Work out the finished part from the listing and answer in its coordinate system (mm). A direction names the side the tool comes from. Round coordinates to 2 decimals unless told otherwise and drop trailing zeros. Order: outer loops, then holes, each group sorted by start corner. A loop starts at its lowest first (then second) coordinate and runs counter-clockwise, first axis right, second up. Notation, with made-up numbers: (67.5, 3.25) -> (93.5, 3.25) arc R20 cw to (93.5, 33.25) -> close; hole circle Ø5 at (87.5, 9.25). An arc over 180 degrees is marked (long way). Use one line per item in the form item = value.
```python
from build123d import *

# Parameters (mm, degrees)
SKETCH2_R               = 18
BOSS_EXTRUDE1_DEPTH     = 22
SKETCH3_R               = 18.5
BOSS_EXTRUDE2_DEPTH     = 26.5
SKETCH4_R               = 1.5
CUT_EXTRUDE1_DEPTH      = 6
CIRPATTERN1_COUNT       = 6
SKETCH5_R               = 6
BOSS_EXTRUDE3_DEPTH     = 6
SKETCH6_R               = 3
BOSS_EXTRUDE4_DEPTH     = 15.5
CUT_EXTRUDE2_DEPTH      = 1
CUT_EXTRUDE2_DEPTH_BACK = 12


with BuildPart() as part:
    # Sketch2 → Boss-Extrude1 (new body)
    with BuildSketch(Plane(origin=(0, 0, 0), x_dir=(1, 0, 0), z_dir=(0, 1, 0))):
        Circle(SKETCH2_R)
    extrude(amount=BOSS_EXTRUDE1_DEPTH)

    # Sketch3 → Boss-Extrude2 (add)
    with BuildSketch(Plane(origin=(0, 22, 0), x_dir=(1, 0, 0), z_dir=(0, 1, 0))):
        Circle(SKETCH3_R)
    extrude(amount=BOSS_EXTRUDE2_DEPTH)

    # Sketch4 → Cut-Extrude1 (cut)
    with BuildSketch(Plane(origin=(0, 48.5, 0), x_dir=(1, 0, 0), z_dir=(0, 1, 0))):
        with Locations((-15.5, 0)):
            Circle(SKETCH4_R)
    cut_extrude1 = extrude(amount=-CUT_EXTRUDE1_DEPTH, mode=Mode.SUBTRACT)

    # CirPattern1: Cut-Extrude1 ×6 about axis
    cirpattern1_axis = Axis((0, 0, 0), (0, 1, 0))
    for i in range(1, CIRPATTERN1_COUNT):
        add(cut_extrude1.rotate(cirpattern1_axis, i * 360 / CIRPATTERN1_COUNT), mode=Mode.SUBTRACT)

    # Sketch5 → Boss-Extrude3 (add)
    with BuildSketch(Plane(origin=(0, 48.5, 0), x_dir=(1, 0, 0), z_dir=(0, 1, 0))):
        with Locations((0, 7)):
            Circle(SKETCH5_R)
    extrude(amount=BOSS_EXTRUDE3_DEPTH)

    # Sketch6 → Boss-Extrude4 (add)
    with BuildSketch(Plane(origin=(0, 54.5, 0), x_dir=(1, 0, 0), z_dir=(0, 1, 0))):
        with Locations((0, 7)):
            Circle(SKETCH6_R)
    extrude(amount=BOSS_EXTRUDE4_DEPTH)

    # Sketch7 → Cut-Extrude2 (cut, two sides)
    with BuildSketch(Plane(origin=(0, 70, 0), x_dir=(1, 0, 0), z_dir=(0, 1, 0))) as cut_extrude2_sk:
        Polygon((-80.661403086, 9.5), (-1.6583, 9.5), (1.6583, 9.5), (80.661403086, 9.5), (80.661403086, 167.506206173), (-80.661403086, 167.506206173), align=None)
    extrude(amount=CUT_EXTRUDE2_DEPTH, mode=Mode.SUBTRACT)
    extrude(cut_extrude2_sk.sketch, amount=-CUT_EXTRUDE2_DEPTH_BACK, mode=Mode.SUBTRACT)


solid = part.part
```
Item 1: The part is cut by section B-B, the plane z = 0. Give the vertices of the cut face in (x, y).
Findings:
outline = (-18.5, 22) -> (-18, 22) -> (-18, 0) -> (18, 0) -> (18, 22) -> (18.5, 22) -> (18.5, 48.5) -> (17, 48.5) -> (17, 42.5) -> (14, 42.5) -> (14, 48.5) -> (-14, 48.5) -> (-14, 42.5) -> (-17, 42.5) -> (-17, 48.5) -> (-18.5, 48.5) -> close
Item 2: The part is cut by section D-D, the plane z = 5. Give the vertices of the cut face in (x, y), and give its area (3 significant figures).
Findings:
outline = (-17.81, 22) -> (-17.29, 22) -> (-17.29, 0) -> (17.29, 0) -> (17.29, 22) -> (17.81, 22) -> (17.81, 48.5) -> (-17.81, 48.5) -> close
area = 1,700 mm^2
Item 3: Consider line 1 along Z through (x, y) = (-7.75, 44); line 2 along Y through (x, z) = (7, 9); line 3 along Y through (x, z) = (-12, -14). Determine where each line is inside the solid, lowest interval first.
Findings:
line_1 = -16.8 to -14.92, -11.92 to 11.92, 14.92 to 16.8
line_2 = 0 to 48.5
line_3 = 22 to 48.5
Item 4: Determine the mould class of faces 6 (the cylindrical face through (17, 46, 0)), 7 (the cylindrical face through (-0.78, 51.46, -12.95)), 8 (the flat face through (4.02, 22, 17.73)) for opening direction X: released by +X, released by -X, zero draft, split by the parting line, or undercut.
Findings:
face_6 = undercut
face_7 = split by the parting line
face_8 = zero draft
Item 5: The part is cut by section A-A, the plane x = 0. Give the vertices of the cut face in (y, z), and give its area (3 significant figures).
Findings:
outline = (0, -18) -> (22, -18) -> (22, -18.5) -> (48.5, -18.5) -> (48.5, -13) -> (54.5, -13) -> (54.5, -10) -> (58, -10) -> (58, -9.5) -> (70, -9.5) -> (70, -4) -> (54.5, -4) -> (54.5, -1) -> (48.5, -1) -> (48.5, 18.5) -> (22, 18.5) -> (22, 18) -> (0, 18) -> close
area = 1,930 mm^2
Item 6: The part is cut by section C-C, the plane y = 59.5. Give the vertices of the cut face in (x, z), and give its area (3 significant figures).
Findings:
outline = (-1.66, -9.5) -> (1.66, -9.5) arc R3 ccw (long way) to start
area = 27.1 mm^2
Item 7: For faces 1 (the flat face through (0, 64, -9.5)), 2 (the flat face through (-8, 42.5, -13)), 3 (the cylindrical face through (-4.01, 35.06, 18.06)), 4 (the cylindrical face through (-2.343, 10.846, -17.847)), 5 (the flat face through (0, 0, 0)), determine the directions among +Z, -Z, +X, -X, +Y, -Y from which every point of the face is accessible in a straight line to the end or side of a thin tool.
Findings:
face_1 = -Z, +X, -X, +Y
face_2 = +Y
face_3 = +Y, -Y
face_4 = -Y
face_5 = +Z, -Z, +X, -X, -Y
Item 8: Flat-ended cylindrical pins translate along their axes: P1, Ø0.9, axis at x = -8, z = -13, coming from the +Y side; P2, Ø8, axis at x = 7.5, z = 0, coming from the +Y side; P3, Ø1, axis at x = 0.5, y = 65.5, coming from the -Z side. Find the tip coordinate at first contact, or state that the pin passes through.
Findings:
P1 = 42.5
P2 = 48.5
P3 = -9.5
